Source: CAD feature listing. Evaluate the final solid. Frame: model axes, mm. A direction names the side the tool comes from. Round coordinates to 2 decimals unless told otherwise and drop trailing zeros. Write each loop counter-clockwise with the first axis right and the second up, starting at its lowest first coordinate (ties: lowest second). Pieces come first, ordered by that corner, then holes. Notation, with made-up numbers: M 66.5,16 L 103.5,16 A27 cw 103.5,49 Z; hole C 12,-10 d2. An arc over 180 degrees is marked long. Answer in a Markdown table with one row per item.
from build123d import *
from build123d.topology import SkipClean

# Parameters (mm, degrees)
BOSS_EXTRU_1_DEPTH      = 5
ESQUISSE2_R             = 1.5
BOSS_EXTRU_2_DEPTH      = 7
ENL_V_MAT_EXTRU_1_DEPTH = 3


with BuildPart() as part:
    # Esquisse1 → Boss.-Extru.1 (new body)
    with BuildSketch(Plane.XY):
        with BuildLine():
            Line((-1.299038106, 0.75), (1.299038106, 0.75))
            ThreePointArc((1.299038106, 0.75), (0, -1.5), (-1.299038106, 0.75))
        make_face()
    extrude(amount=BOSS_EXTRU_1_DEPTH)

    # Esquisse2 → Boss.-Extru.2 (add)
    with SkipClean():  # the faces are left unmerged after this step: merging them gives an invalid solid
        with BuildSketch(Plane.XY.offset(5)):
            with Locations(Location((0, 0, 0), (0, 0, 150))):
                Circle(ESQUISSE2_R)
        extrude(amount=BOSS_EXTRU_2_DEPTH)

    # Esquisse3 → Enlèv. mat.-Extru.1 (cut)
    with SkipClean():  # the faces are left unmerged after this step: merging them gives an invalid solid
        with BuildSketch(Plane(origin=(1.5, 0, 0), x_dir=(0, 0, -1), z_dir=(1, 0, 0))):
            with BuildLine():
                Line((-8, 1.5), (-5, 1.5))
                Line((-5, 1.5), (-5, 0.75))
                add(Edge.make_bspline(
                    [(-8, 1.5), (-6.894526205, 0.811843176), (-5, 0.75)],
                    knots=[0, 0, 0, 0.697141836, 0.697141836, 0.697141836], degree=2))
            make_face()
        extrude(amount=-ENL_V_MAT_EXTRU_1_DEPTH, mode=Mode.SUBTRACT)


solid = part.part
Q1. Material intervals for probe 1 along Y at (x, z) = (0.05, 3.5); probe 2 along X at (y, z) = (-0.3, 4.25); probe 3 along Y at (x, z) = (-0.5, 6.5), sorted ascending.
Solutions:
| item | result |
|---|---|
| probe 1 | y = -1.5 to 0.75 |
| probe 2 | x = -1.47 to 1.47 |
| probe 3 | y = -1.41 to 0.92 |
Q2. Access query for faces 1 (the flat face through (0, 0.75, 2)), 2 (the flat face through (0, 0, 12)). Directions: +Z, -Z, +X, -X, +Y, -Y. A direction counts if a zero-diameter tool reaches every point of the face in a straight line with its end or side. Return the directions, or none.
Solutions:
| item | result |
|---|---|
| face 1 | -Z, +X, -X, +Y |
| face 2 | +Z, +X, -X, +Y, -Y |
Q3. Section A-A (y = -0.7). Return loops of the section in (x, z).
Solutions:
| item | result |
|---|---|
| outline | M -1.33,0 L 1.33,0 L 1.33,12 L -1.33,12 Z |
Q4. Section C-C (z = 1). Return loops of the section in (x, y), and give its area (3 significant figures).
Solutions:
| item | result |
|---|---|
| outline | M -1.3,0.75 A1.5 ccw long 1.3,0.75 Z |
| area | 5.69 mm2 |
Q5. Section B-B (z = 9.75). Return loops of the section in (x, y).
Solutions:
| item | result |
|---|---|
| outline | C 0,0 d3 |
Q6. Section D-D (y = -1.2). Return loops of the section in (x, z), and give its area (3 significant figures).
Solutions:
| item | result |
|---|---|
| outline | M -0.9,0 L 0.9,0 L 0.9,12 L -0.9,12 Z |
| area | 21.6 mm2 |
